Can you work these out from the model? Positions are in its coordinate system, mm. A direction names the side the tool comes from. Give positions to 0.01 mm unless a question says otherwise; leave off trailing zeros. Order: outer loops, then holes, each group sorted by start corner. A loop starts at its lowest first (then second) coordinate and runs counter-clockwise, first axis right, second up. Notation, with made-up numbers: M -1,54.25 L 37,54.25 A25 cw 37,73.25 Z; hole C 18,-4.5 d1. An arc over 180 degrees is marked long. Use a Markdown table: item, result. Add a question column.
from build123d import *

# Parameters (mm, degrees)
F0_R     = 1.5
F1_DEPTH = 2
F2_R     = 1.99999


# Not quite as in the source:
# - a fillet or chamfer is up to 0.001 mm smaller than in the source, because OpenCascade refuses the exact size


with BuildPart() as f1:
    # F0 (on Top) → F1 (new body)
    with BuildSketch(Plane.XY):
        Polygon((10.5, 31.5), (-10.5, 31.5), (-10.5, 27.5), (-18, 27.5), (-18, 21.5), (-23, 21.5), (-23, -31.5), (23, -31.5), (23, 21.5), (18, 21.5), (18, 27.5), (10.5, 27.5), align=None)
        with Locations((-15, -20.5)):
            Circle(F0_R, mode=Mode.SUBTRACT)
        with Locations((15.5, -20.5)):
            Circle(F0_R, mode=Mode.SUBTRACT)
        with Locations((-15, 10)):
            Circle(F0_R, mode=Mode.SUBTRACT)
        with Locations((15.5, 10)):
            Circle(F0_R, mode=Mode.SUBTRACT)
    extrude(amount=F1_DEPTH)

    # F2 (radius 2 in the source; OpenCascade refuses exactly that, so slightly less here)
    f2_edges = [f1.edges().sort_by_distance(p)[0] for p in [
        (10.5, 31.5, 1),
        (23, 21.5, 1),
        (18, 27.5, 1),
        (18, 21.5, 1),
        (10.5, 27.5, 1),
        (-10.5, 31.5, 1),
        (-10.5, 27.5, 1),
        (-18, 27.5, 1),
        (-18, 21.5, 1),
        (-23, 21.5, 1),
        (-23, -31.5, 1),
        (23, -31.5, 1),
    ]]
    fillet(f2_edges, radius=F2_R)


solid = f1.part
1. On a 3-axis mill with a long thin cutter (end or side, diameter ignored), from which of +Z, -Z, +X, -X, +Y, -Y can I reach the whole of each face in a straight line? I mean faces 4 (the face through (-23, -5, 1)), 5 (the face through (14, 27.5, 1)), 6 (the face through (-18, 25, 1)). Say none if no direction works.
2. We'd pull the mould along X, two halves only. Please class faces 1 (the face through (-16.5, 10.07, 0.99)), 2 (the face through (0, 0, 2)), 3 (the face through (18, 24, 1)): +X half, -X half, draft (parallel to the pull), parting line (faces both ways), or undercut.
3. If we section it at A-A, the plane x = -15: List the corners of the cut face in (y, z) for me.
4. Will these pins go through, and if not, where does the flat tip stop? pin 1 (0.5 mm diameter, centred on x = -20.5, z = 0.5, fed in from +Y); pin 2 (0.6 mm diameter, centred on x = -14, z = 1, fed in from +Y); pin 3 (0.6 mm diameter, centred on y = 24.5, z = 1, fed in from -X).
5. If we section it at C-C, the plane z = 0.6: State how many separate pieces and enclosed holes the cut face has, then the cut area to 3 significant figures.
6. I need wall thicknesses on L1, parallel to Y at x = -15, z = 0.5; L2, parallel to Y at x = 15, z = 0.65; L3, parallel to X at y = 27, z = 0.4. Which ranges of each line are inside material? Lowest first, please. Write a range as [from, to].
7. If we section it at B-B, the plane y = 10: List the corners of the cut face in (x, z) for me.
Geometry results:
| question | item | result |
|---|---|---|
| 1 | face 4 | +Z, -Z, -X, +Y, -Y |
| 1 | face 5 | +Z, -Z, +X, +Y |
| 1 | face 6 | +Z, -Z, -X, +Y |
| 2 | face 1 | undercut |
| 2 | face 2 | draft |
| 2 | face 3 | +X half |
| 3 | outline | M -31.5,0 L -22,0 L -22,2 L -31.5,2 Z; M -19,0 L 8.5,0 L 8.5,2 L -19,2 Z; M 11.5,0 L 27.5,0 L 27.5,2 L 11.5,2 Z |
| 4 | pin 1 | stops at y = 21.5 |
| 4 | pin 2 | stops at y = 27.5 |
| 4 | pin 3 | stops at x = -18 |
| 5 | separate pieces | 1 |
| 5 | enclosed holes | 4 |
| 5 | area | 2,710 mm^2 |
| 6 | L1 | y = [-31.5, -22], [-19, 8.5], [11.5, 27.5] |
| 6 | L2 | y = [-31.5, -21.91], [-19.09, 8.59], [11.41, 27.5] |
| 6 | L3 | x = [-17.32, 17.32] |
| 7 | outline | M -23,0 L -16.5,0 L -16.5,2 L -23,2 Z; M -13.5,0 L 14,0 L 14,2 L -13.5,2 Z; M 17,0 L 23,0 L 23,2 L 17,2 Z |
